```python
from build123d import *

# Parameters (mm, degrees)
SKIZZE1_W                       = 7.62
SKIZZE1_H                       = 2.54
SKIZZE1_W_2                     = 0.7
SKIZZE1_H_2                     = 0.7
AUFSATZ_LINEAR_AUSTRAGEN1_DEPTH = 14
SKIZZE3_OUTSIDE_W               = 12.848
SKIZZE3_OUTSIDE_H               = 7.768
SKIZZE3_OUTSIDE_W_2             = 7.42
SKIZZE3_OUTSIDE_H_2             = 2.34
SCHNITT_LINEAR_AUSTRAGEN1_DEPTH = 9
FASE1_SIZE                      = 0.3
FASE1_SIZE2                     = 1.701384546
FASE1_PART_2_SIZE               = 0.3
FASE1_PART_2_SIZE2              = 1.701384546


with BuildPart() as part:
    # Skizze1 → Aufsatz-Linear austragen1 (new body)
    with BuildSketch(Plane(origin=(0, 0, 0), x_dir=(1, 0, 0), z_dir=(0, 1, 0))):
        Rectangle(SKIZZE1_W, SKIZZE1_H)
        with Locations((-2.54, 0)):
            Rectangle(SKIZZE1_W_2, SKIZZE1_H_2, mode=Mode.SUBTRACT)
        Rectangle(SKIZZE1_W_2, SKIZZE1_H_2, mode=Mode.SUBTRACT)
        with Locations((2.54, 0)):
            Rectangle(SKIZZE1_W_2, SKIZZE1_H_2, mode=Mode.SUBTRACT)
    extrude(amount=AUFSATZ_LINEAR_AUSTRAGEN1_DEPTH)

    # Skizze3 outside → Schnitt-Linear austragen1 (cut)
    with BuildSketch(Plane.XZ):
        Rectangle(SKIZZE3_OUTSIDE_W, SKIZZE3_OUTSIDE_H)
        Rectangle(SKIZZE3_OUTSIDE_W_2, SKIZZE3_OUTSIDE_H_2, mode=Mode.SUBTRACT)
    extrude(amount=-SCHNITT_LINEAR_AUSTRAGEN1_DEPTH, mode=Mode.SUBTRACT)

    # Fase1
    fase1_edges = [part.edges().sort_by_distance(p)[0] for p in [
        (-2.89, 0, 0),
        (-2.54, 0, 0.35),
        (-2.19, 0, 0),
        (-2.54, 0, -0.35),
        (-0.35, 0, 0),
        (0, 0, 0.35),
        (0.35, 0, 0),
        (0, 0, -0.35),
        (2.19, 0, 0),
        (2.54, 0, 0.35),
        (2.89, 0, 0),
        (2.54, 0, -0.35),
    ]]
    fase1_side = [part.faces().sort_by_distance(p)[0] for p in [
        (0, 0, -1.092197686),
    ]]
    chamfer(fase1_edges, length=FASE1_SIZE, length2=FASE1_SIZE2, reference=fase1_side[0])

    # Fase1 part 2
    fase1_part_2_edges = [part.edges().sort_by_distance(p)[0] for p in [
        (-2.89, 14, 0),
        (-2.54, 14, 0.35),
        (-2.19, 14, 0),
        (-2.54, 14, -0.35),
        (-0.35, 14, 0),
        (0, 14, 0.35),
        (0.35, 14, 0),
        (0, 14, -0.35),
        (2.19, 14, 0),
        (2.54, 14, 0.35),
        (2.89, 14, 0),
        (2.54, 14, -0.35),
    ]]
    fase1_part_2_side = [part.faces().sort_by_distance(p)[0] for p in [
        (0, 14, 1.189678147),
    ]]
    chamfer(fase1_part_2_edges, length=FASE1_PART_2_SIZE, length2=FASE1_PART_2_SIZE2, reference=fase1_part_2_side[0])


solid = part.part
```
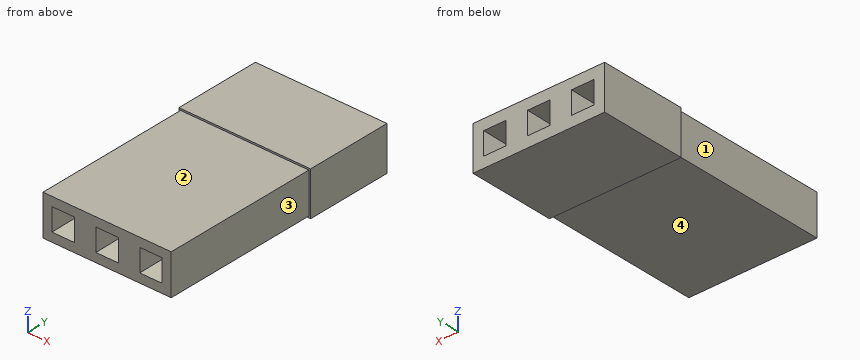
For this review, take the finished solid that the model builds, in its own axes (mm). Face numbers are marked on the shaded views. A direction names the side the tool comes from. Coordinates: 2 decimals unless noted, no trailing zeros. Write each loop counter-clockwise with the first axis right and the second up, starting at its lowest first coordinate (ties: lowest second). Pieces come first, ordered by that corner, then holes. Notation, with made-up numbers: (71.25, 14) - (97.25, 14) arc R35 ccw to (97.25, 53) - close; hole circle Ø7 at (-12.5, 30.25). An arc over 180 degrees is marked (long way). Answer in a Markdown table with one row per item. Add a question column.
Q1. For P1, Ø0.6, axis at y = 6.5, z = 0, coming from the +X side; P2, Ø0.8, axis at y = 8, z = 0, coming from the -X side, all flat-tipped, find the tip position at first contact; note any pin that passes through.
Q2. Tool access review of the marked faces 1, 2, 3 and 4: name each direction out of +Z, -Z, +X, -X, +Y, -Y from which nothing blocks a thin tool from reaching the whole face with its end or side.
Q3. We need section C-C, the plane x = -2.5. State the section outline as (y, z) points, and give its area (3 significant figures).
Q4. We need section A-A, the plane z = 0.15. Count the separate pieces of the cut face and the enclosed holes in it, and give its area (3 significant figures).
Q5. We need section B-B, the plane y = 11.75. State the section outline as (x, z) points, and give its area (3 significant figures).
Q6. For probe 1 along X at (y, z) = (6.25, 0.15); probe 2 along Z at (x, y) = (-2.25, 3.25), list the stretches that pass through material, from the lowest coordinate up.
Q7. We need section D-D, the plane z = 0.8. State the section outline as (x, y) points.
Answer list:
| question | item | result |
|---|---|---|
| 1 | P1 | stops at x = 3.71 |
| 1 | P2 | stops at x = -3.71 |
| 2 | face 1 | +Z, -Z, -X, -Y |
| 2 | face 2 | +Z, +X, -X, -Y |
| 2 | face 3 | +Z, -Z, +X, -Y |
| 2 | face 4 | -Z, +X, -X, -Y |
| 3 | outline | (0, -1.17) - (9, -1.17) - (9, -1.27) - (14, -1.27) - (14, -0.65) - (12.3, -0.35) - (1.7, -0.35) - (0, -0.65) - close; (0, 0.65) - (1.7, 0.35) - (12.3, 0.35) - (14, 0.65) - (14, 1.27) - (9, 1.27) - (9, 1.17) - (0, 1.17) - close |
| 3 | area | 22.9 mm2 |
| 4 | separate pieces | 4 |
| 4 | enclosed holes | 0 |
| 4 | area | 72.4 mm2 |
| 5 | outline | (-3.81, -1.27) - (3.81, -1.27) - (3.81, 1.27) - (-3.81, 1.27) - close; hole (-2.89, -0.35) - (-2.19, -0.35) - (-2.19, 0.35) - (-2.89, 0.35) - close; hole (-0.35, -0.35) - (0.35, -0.35) - (0.35, 0.35) - (-0.35, 0.35) - close; hole (2.19, -0.35) - (2.89, -0.35) - (2.89, 0.35) - (2.19, 0.35) - close |
| 5 | area | 17.9 mm2 |
| 6 | probe 1 | x = -3.71 to -2.89, -2.19 to -0.35, 0.35 to 2.19, 2.89 to 3.71 |
| 6 | probe 2 | z = -1.17 to -0.35, 0.35 to 1.17 |
| 7 | outline | (-3.81, 9) - (-3.71, 9) - (-3.71, 0) - (3.71, 0) - (3.71, 9) - (3.81, 9) - (3.81, 14) - (-3.81, 14) - close |
